Could you check a few things on this model? Use its own coordinates, in mm. Coordinates: 2 decimals unless noted, no trailing zeros. Write each loop counter-clockwise with the first axis right and the second up, starting at its lowest first coordinate (ties: lowest second). Pieces come first, ordered by that corner, then holes. Notation, with made-up numbers: M 48,74 L 74,74 A32 ccw 74,112 Z; hole C 24.25,-21 d8. An arc over 180 degrees is marked long. Write item = value, one per line.
```python
from build123d import *

# Parameters (mm, degrees)
F1_DEPTH = 177.8
F3_DEPTH = 25.4


# Not quite as in the source:
# - a feature names something its author has since deleted; it is built from what else it names


with BuildPart() as f1:
    # F0 (on Front) → F1 (new body)
    with BuildSketch(Plane.XZ):
        Polygon((0, 1.9812), (0, 0), (19.05, 0), (23.8252, 1.9812), align=None)
        Polygon((-19.05, 0), (0, 0), (0, 1.9812), (-23.8252, 1.9812), align=None)
    extrude(amount=F1_DEPTH)

    # F2 (on Right) → F3 (cut, symmetric)
    with BuildSketch(Plane.YZ):
        Polygon((-177.7999848127, 1.9810541999), (0, 0), (0, 5.3311795928), (-177.7999848127, 1.9878952298), align=None)
    extrude(amount=F3_DEPTH, both=True, mode=Mode.SUBTRACT)


solid = f1.part
```
Item 1: I'm going to push flat-ended pins straight in: P1, Ø6, axis at x = -2, y = -140.5, coming from the +Z side; P2, Ø3, axis at x = -11, y = -156, coming from the -Z side; P3, Ø1.5, axis at x = -10.5, y = -51.5, coming from the +Z side. Where does each tip first touch, or does it pass through?
Numbers:
P1 = 1.6
P2 = 0
P3 = 0.58
Item 2: Imagine slicing it at C-C (y = -75). Write out the boundary of the cut face in (x, z), and give its area (3 significant figures).
Numbers:
outline = M -21.06,0.84 L -19.05,0 L 19.05,0 L 21.06,0.84 Z
area = 33.5 mm²
Item 3: If I drill on line 1 along X through (y, z) = (-123, 0.3); line 2 along Z through (x, y) = (17, -127.5); line 3 along X through (y, z) = (-140, 0.5), over which ranges is the centre line in solid material (lowest first)?
Numbers:
line_1 = -19.77 to 19.77
line_2 = 0 to 1.42
line_3 = -20.26 to 20.26
Item 4: Imagine slicing it at B-B (z = 1.6). Write out the boundary of the cut face in (x, y).
Numbers:
outline = M -22.91,-177.8 L 22.91,-177.8 L 22.91,-143.6 L -22.91,-143.6 Z
